Can you work these out from the model? Positions are in its coordinate system, mm. A direction names the side the tool comes from. Give positions to 0.01 mm unless a question says otherwise; leave off trailing zeros. Write each loop counter-clockwise with the first axis right and the second up, starting at its lowest first coordinate (ties: lowest second). Pieces come first, ordered by that corner, then holes.
```python
from build123d import *

# Parameters (mm, degrees)
SKETCH4_W           = 21
SKETCH4_H           = 4
BOSS_EXTRUDE3_DEPTH = 19
SKETCH3_R           = 1.025
BOSS_EXTRUDE2_DEPTH = 4
SKETCH7_R           = 2
CUT_EXTRUDE2_DEPTH  = 2.5
SKETCH6_R           = 4
CUT_EXTRUDE1_DEPTH  = 39.474017206
FILLET2_R           = 5
FILLET3_R           = 5
FILLET4_R           = 2


with BuildPart() as part:
    # Sketch4 → Boss-Extrude3 (new, symmetric)
    with BuildSketch(Plane.XY):
        Rectangle(SKETCH4_W, SKETCH4_H)
    extrude(amount=BOSS_EXTRUDE3_DEPTH, both=True)

    # Sketch3 → Boss-Extrude2 (add)
    with BuildSketch(Plane.XY.offset(19)):
        with BuildLine():
            Line((10.5, -27), (10.5, 2))
            Line((10.5, 2), (-10.5, 2))
            Line((-10.5, 2), (-10.5, -27))
            Line((-10.5, -27), (-3.676525192, -27))
            ThreePointArc((-3.676525192, -27), (-3.995419387, -22.334749823), (0, -19.905166188))
            ThreePointArc((0, -19.905166188), (3.995419387, -22.334749823), (3.676525192, -27))
            Line((3.676525192, -27), (10.5, -27))
        make_face()
        with Locations((-7.999402765, -24.502917938)):
            Circle(SKETCH3_R, mode=Mode.SUBTRACT)
        with Locations((-5.636784611, -18.799053148)):
            Circle(SKETCH3_R, mode=Mode.SUBTRACT)
        with Locations((8.133563123, -24.502917938)):
            Circle(SKETCH3_R, mode=Mode.SUBTRACT)
        with Locations((0.067080179, -16.436434994)):
            Circle(SKETCH3_R, mode=Mode.SUBTRACT)
        with Locations((5.770944969, -18.799053148)):
            Circle(SKETCH3_R, mode=Mode.SUBTRACT)
    boss_extrude2 = extrude(amount=BOSS_EXTRUDE2_DEPTH)

    # Sketch7 → Cut-Extrude2 (cut)
    with BuildSketch(Plane.XY.offset(23)):
        with Locations((-7.999402765, -24.502917938)):
            Circle(SKETCH7_R)
        with Locations((-5.636784611, -18.799053148)):
            Circle(SKETCH7_R)
        with Locations((0.067080179, -16.436434994)):
            Circle(SKETCH7_R)
        with Locations((5.770944969, -18.799053148)):
            Circle(SKETCH7_R)
        with Locations((8.133563123, -24.502917938)):
            Circle(SKETCH7_R)
    cut_extrude2 = extrude(amount=-CUT_EXTRUDE2_DEPTH, mode=Mode.SUBTRACT)

    # Mirror1: Boss-Extrude2, Cut-Extrude2 across plane
    add(boss_extrude2.mirror(Plane.XY))
    add(cut_extrude2.mirror(Plane.XY), mode=Mode.SUBTRACT)

    # Sketch6 → Cut-Extrude1 (cut, through all)
    with BuildSketch(Plane(origin=(0, 2, 0), x_dir=(1, 0, 0), z_dir=(0, 1, 0))):
        with Locations(Location((0, 0, 0), (0, 0, 270))):
            Circle(SKETCH6_R)
        with BuildLine():
            ThreePointArc((0, 9.025), (-1.025, 8), (0, 6.975))
            ThreePointArc((0, 6.975), (1.025, 8), (0, 9.025))
        make_face()
        with BuildLine():
            ThreePointArc((-6, 10.75), (-4.75, 12), (-6, 13.25))
            ThreePointArc((-6, 13.25), (-7.25, 12), (-6, 10.75))
        make_face()
        with BuildLine():
            ThreePointArc((-2.25, 8), (-3.5, 9.25), (-4.75, 8))
            ThreePointArc((-4.75, 8), (-3.5, 6.75), (-2.25, 8))
        make_face()
        with BuildLine():
            ThreePointArc((-5.656854249, 4.631854249), (-4.631854249, 5.656854249), (-5.656854249, 6.681854249))
            ThreePointArc((-5.656854249, 6.681854249), (-6.681854249, 5.656854249), (-5.656854249, 4.631854249))
        make_face()
        with BuildLine():
            ThreePointArc((-8, 2.475), (-6.975, 3.5), (-8, 4.525))
            ThreePointArc((-8, 4.525), (-9.025, 3.5), (-8, 2.475))
        make_face()
        with BuildLine():
            ThreePointArc((-2.475, -8), (-3.5, -6.975), (-4.525, -8))
            ThreePointArc((-4.525, -8), (-3.5, -9.025), (-2.475, -8))
        make_face()
        with BuildLine():
            ThreePointArc((0, -6.975), (-1.025, -8), (0, -9.025))
            ThreePointArc((0, -9.025), (1.025, -8), (0, -6.975))
        make_face()
        with BuildLine():
            ThreePointArc((-8, -1.025), (-6.975, 0), (-8, 1.025))
            ThreePointArc((-8, 1.025), (-9.025, 0), (-8, -1.025))
        make_face()
        with BuildLine():
            ThreePointArc((-8, -4.75), (-6.75, -3.5), (-8, -2.25))
            ThreePointArc((-8, -2.25), (-9.25, -3.5), (-8, -4.75))
        make_face()
        with BuildLine():
            ThreePointArc((-5.656854249, -6.681854249), (-4.631854249, -5.656854249), (-5.656854249, -4.631854249))
            ThreePointArc((-5.656854249, -4.631854249), (-6.681854249, -5.656854249), (-5.656854249, -6.681854249))
        make_face()
        with BuildLine():
            ThreePointArc((-6, -13.25), (-4.75, -12), (-6, -10.75))
            ThreePointArc((-6, -10.75), (-7.25, -12), (-6, -13.25))
        make_face()
        with BuildLine():
            ThreePointArc((6, 13.25), (4.75, 12), (6, 10.75))
            ThreePointArc((6, 10.75), (7.25, 12), (6, 13.25))
        make_face()
        with BuildLine():
            ThreePointArc((2.475, 8), (3.5, 6.975), (4.525, 8))
            ThreePointArc((4.525, 8), (3.5, 9.025), (2.475, 8))
        make_face()
        with BuildLine():
            ThreePointArc((5.656854249, 4.631854249), (6.681854249, 5.656854249), (5.656854249, 6.681854249))
            ThreePointArc((5.656854249, 6.681854249), (4.631854249, 5.656854249), (5.656854249, 4.631854249))
        make_face()
        with BuildLine():
            ThreePointArc((8, 2.25), (9.25, 3.5), (8, 4.75))
            ThreePointArc((8, 4.75), (6.75, 3.5), (8, 2.25))
        make_face()
        with BuildLine():
            ThreePointArc((8, -1.025), (9.025, 0), (8, 1.025))
            ThreePointArc((8, 1.025), (6.975, 0), (8, -1.025))
        make_face()
        with BuildLine():
            ThreePointArc((8, -4.525), (9.025, -3.5), (8, -2.475))
            ThreePointArc((8, -2.475), (6.975, -3.5), (8, -4.525))
        make_face()
        with BuildLine():
            ThreePointArc((5.656854249, -6.681854249), (6.681854249, -5.656854249), (5.656854249, -4.631854249))
            ThreePointArc((5.656854249, -4.631854249), (4.631854249, -5.656854249), (5.656854249, -6.681854249))
        make_face()
        with BuildLine():
            ThreePointArc((2.25, -8), (3.5, -9.25), (4.75, -8))
            ThreePointArc((4.75, -8), (3.5, -6.75), (2.25, -8))
        make_face()
        with BuildLine():
            ThreePointArc((6, -13.25), (7.25, -12), (6, -10.75))
            ThreePointArc((6, -10.75), (4.75, -12), (6, -13.25))
        make_face()
    extrude(amount=-CUT_EXTRUDE1_DEPTH, mode=Mode.SUBTRACT)

    # Fillet2
    fillet2_edges = [part.edges().sort_by_distance(p)[0] for p in [
        (0, -2, 19),
        (0, -2, -19),
    ]]
    fillet(fillet2_edges, radius=FILLET2_R)

    # Fillet3
    fillet3_edges = [part.edges().sort_by_distance(p)[0] for p in [
        (0, 2, 23),
        (0, 2, -23),
    ]]
    fillet(fillet3_edges, radius=FILLET3_R)

    # Fillet4
    fillet4_edges = [part.edges().sort_by_distance(p)[0] for p in [
        (-10.5, -27, 21),
        (-3.676525192, -27, 21),
        (3.676525192, -27, 21),
        (10.5, -27, 21),
        (-3.676525192, -27, -21),
        (-10.5, -27, -21),
        (10.5, -27, -21),
        (3.676525192, -27, -21),
    ]]
    fillet(fillet4_edges, radius=FILLET4_R)


solid = part.part
```
1) If we mould it in two halves opening along Y, with no side actions, what happens to faces 1 (the face through (-8, -27, -21)), 2 (the face through (-4.656, 0.028, -5.435)), 3 (the face through (-8.222, -25.504, -19.74))? For each: +Y half, -Y half, draft (parallel to the pull), parting line (faces both ways), or undercut.
Values follow:
face 1: -Y half
face 2: draft
face 3: undercut
2) Suppose I cut it at A-A on y = -10.5. Write out the boundary of the cut face in (x, z).
Values follow:
outline: (-10.5, -23) - (10.5, -23) - (10.5, -19) - (-10.5, -19) - close; (-10.5, 19) - (10.5, 19) - (10.5, 23) - (-10.5, 23) - close
3) For faces 4 (the face through (-7.1, -25.4, -20.5)), 5 (the face through (5.511, -16.816, 21.768)), 6 (the face through (0, -15, -19)), 7 (the face through (0, -12, -23)), 8 (the face through (6.76, 0.03, 12.99)), which set-ups out of +Z, -Z, +X, -X, +Y, -Y let a thin tool reach every point of the face, with its end or its side?
Values follow:
face 4: -Z
face 5: +Z
face 6: +X, -X, -Y
face 7: -Z, +X, -X, +Y, -Y
face 8: +Y, -Y
4) For pin 1 Ø2.5 at (x, y) = (8.13, -24.5) entering from -Z; pin 2 Ø5 at (x, z) = (-1, -14) entering from -Y; pin 3 Ø2 at (x, y) = (5, -19) entering from +Z; pin 4 Ø6 at (y, z) = (-6.5, 9) entering from +X, each with a flat end and sliding along its axis, tell me the tip position at first contact or that it passes through.
Values follow:
pin 1: stops at z = -20.5
pin 2: stops at y = -2.67
pin 3: stops at z = 20.5
pin 4: passes through
5) Suppose I cut it at B-B on y = -23. State how many separate pieces and enclosed holes the cut face has, plus the area to 3 significant figures.
Values follow:
separate pieces: 4
enclosed holes: 0
area: 73.2 mm2
6) Please list where these lines run through material, in increasing order: L1, parallel to X at y = 0.75, z = 0 (3 decimals); L2, parallel to Z at x = 8, y = -18.5; L3, parallel to Z at x = 6.5, y = 0.
Values follow:
L1: x = -10.5 to -9.025, -6.975 to -4, 4 to 6.975, 9.025 to 10.5
L2: z = -23 to -19, 19 to 23
L3: z = -22 to -13.15, -10.85 to -6.24, -5.07 to 5.07, 6.24 to 10.85, 13.15 to 22
